from build123d import *

# Parameters (mm, degrees)
F0_R     = 5.65
F0_R_2   = 4.3
F1_DEPTH = 0.7
F0_R_3   = 6.35
F2_DEPTH = 10


with BuildPart() as f1:
    # F0 (on Top) → F1 (new body)
    with BuildSketch(Plane.XY):
        Circle(F0_R)
        Circle(F0_R_2, mode=Mode.SUBTRACT)
    extrude(amount=F1_DEPTH)

    # F0 (on Top) → F2 (join)
    with BuildSketch(Plane.XY):
        Circle(F0_R_3)
        Circle(F0_R, mode=Mode.SUBTRACT)
        Circle(F0_R)
        Circle(F0_R_2, mode=Mode.SUBTRACT)
    extrude(amount=-F2_DEPTH)


solid = f1.part
Source: CAD feature listing. Evaluate the final solid. Frame: model axes, mm. A direction names the side the tool comes from. Round coordinates to 2 decimals unless told otherwise and drop trailing zeros. Loops run counter-clockwise (first coordinate to the right, second up) from the corner with the lowest first, then second, coordinate; pieces in that order, holes last. Notation, with made-up numbers: (-16.5, 45.5) - (-1.5, 45.5) arc R23 ccw to (-1.5, 75.5) - close; hole circle Ø8 at (27, 41.25). An arc over 180 degrees is marked (long way). Write item = value, one per line. Start each with the question number.
(1) Ray query, line 1 along Y through (x, z) = (0, -5.5); line 2 along X through (y, z) = (0.75, -4); line 3 along Z through (x, y) = (-4.75, 3.5). Return the intervals inside material, ascending. Write a range as from..to.
(2) Set-up query: faces 1 (the face through (-2, -4, -10)), 2 (the face through (-6, 0, 0)). Return all of +Z, -Z, +X, -X, +Y, -Y with unobstructed straight access to the full face (end or side cutting, diameter ignored); none if empty.
(3) Section query A-A, the plane x = 0. Output: boundary loops of the cut face in (y, z).
(4) Pin query (flat end, axial travel): pin 1 (4 mm diameter, centred on x = 2.5, z = -4.5, fed in from -Y); pin 2 (6 mm diameter, centred on y = 5, z = -4.5, fed in from +X). Return the tip coordinate at first contact, or that it passes through.
(5) Section query C-C, the plane z = -6.5. Output: boundary loops of the cut face in (x, y).
Conclusion:
q1.line_1 = -6.35..-4.3, 4.3..6.35
q1.line_2 = -6.31..-4.23, 4.23..6.31
q1.line_3 = -10..0
q2.face_1 = -Z, +X, -X, +Y, -Y
q2.face_2 = +Z
q3.outline = (-6.35, -10) - (-4.3, -10) - (-4.3, 0.7) - (-5.65, 0.7) - (-5.65, 0) - (-6.35, 0) - close; (4.3, -10) - (6.35, -10) - (6.35, 0) - (5.65, 0) - (5.65, 0.7) - (4.3, 0.7) - close
q4.pin_1 = -6.33
q4.pin_2 = 6.03
q5.outline = circle Ø12.7 at (0, 0); hole circle Ø8.6 at (0, 0)
